```python
from build123d import *

# Parameters (mm, degrees)
F0_R     = 27.178
F0_R_2   = 24.638
F1_DEPTH = 27.813
F0_R_3   = 30.353
F2_DEPTH = 3.175
F3_R     = 2.54
F4_SIZE  = 1.905


with BuildPart() as f1:
    # F0 (on Front) → F1 (new body)
    with BuildSketch(Plane.XZ):
        Circle(F0_R)
        Circle(F0_R_2, mode=Mode.SUBTRACT)
    extrude(amount=F1_DEPTH)

    # F0 (on Front) → F2 (join)
    with BuildSketch(Plane.XZ):
        Circle(F0_R_3)
        Circle(F0_R, mode=Mode.SUBTRACT)
    extrude(amount=F2_DEPTH)

    # F3
    f3_edges = [f1.edges().sort_by_distance(p)[0] for p in [
        (-24.638, 0, 0),
    ]]
    fillet(f3_edges, radius=F3_R)

    # F4
    f4_edges = [f1.edges().sort_by_distance(p)[0] for p in [
        (-30.353, 0, 0),
    ]]
    chamfer(f4_edges, length=F4_SIZE)


solid = f1.part
```
The listing builds one solid part. Answer for the finished solid, in the listing's coordinates (mm). A direction names the side the tool comes from. Give positions to 0.01 mm unless a question says otherwise; leave off trailing zeros. Loops run counter-clockwise (first coordinate to the right, second up) from the corner with the lowest first, then second, coordinate; pieces in that order, holes last. Notation, with made-up numbers: M 88.5,37 L 103.5,37 A34 cw 103.5,71 Z; hole C 69,-16 d10. An arc over 180 degrees is marked long. One line per item, written item: value.
1. Section A-A on x = 0 is taken. Determine the outline of the cut face in (y, z) (3 decimals).
Found:
outline: M -27.813,-27.178 L -3.175,-27.178 L -3.175,-30.353 L -1.905,-30.353 L 0,-28.448 L 0,-27.178 A2.54 ccw -2.54,-24.638 L -27.813,-24.638 Z; M -27.813,24.638 L -2.54,24.638 A2.54 ccw 0,27.178 L 0,28.448 L -1.905,30.353 L -3.175,30.353 L -3.175,27.178 L -27.813,27.178 Z
2. Find the intervals of material crossed by probe 1 along Z at (x, y) = (0, -22); probe 2 along Z at (x, y) = (8, -22.75); probe 3 along X at (y, z) = (-26.25, 7), in increasing order.
Found:
probe 1: -27.18 to -24.64, 24.64 to 27.18
probe 2: -25.97 to -23.3, 23.3 to 25.97
probe 3: -26.26 to -23.62, 23.62 to 26.26
3. For faces 4 (the face through (-23, -3.175, -16)), 5 (the face through (23, 0, -15)), determine the directions among +Z, -Z, +X, -X, +Y, -Y from which every point of the face is accessible in a straight line to the end or side of a thin tool.
Found:
face 4: -Y
face 5: +Z, -Z, +X, -X, +Y
4. Section C-C on y = -23 is taken. Determine the outline of the cut face in (x, z), plus the area to 3 significant figures.
Found:
outline: C 0,0 d54.36; hole C 0,0 d49.28
area: 413 mm^2
5. Each of these flat-tipped pins is pushed along its axis until it touches: P1, Ø12, axis at x = 2, y = -14, coming from the +Z side; P2, Ø8, axis at y = -24, z = 21, coming from the +X side; P3, Ø10, axis at x = 7, y = -19, coming from the -Z side. Where does it stop, or does it pass through?
Found:
P1: z = 27.18
P2: x = 21.2
P3: z = -27.1
6. For a pull along X with two mould halves and no side action, classify faces 1 (the face through (-6.17, -27.813, -24.03)), 2 (the face through (28.95, -2.53, 9.12)), 3 (the face through (-5.341, -15, -24.052)) as pulls with the +X half, pulls with the -X half, needs draft (parallel to the pull), parting line crosses it, or undercut.
Found:
face 1: needs draft
face 2: parting line crosses it
face 3: undercut
7. Section B-B on z = 0 is taken. Determine the outline of the cut face in (x, y) (3 decimals).
Found:
outline: M -30.353,-3.175 L -27.178,-3.175 L -27.178,-27.813 L -24.638,-27.813 L -24.638,-2.54 A2.54 ccw -27.178,0 L -28.448,0 L -30.353,-1.905 Z; M 24.638,-27.813 L 27.178,-27.813 L 27.178,-3.175 L 30.353,-3.175 L 30.353,-1.905 L 28.448,0 L 27.178,0 A2.54 ccw 24.638,-2.54 Z
